Job drawing, mm, ordinate dimensions from the low corner. One solid piece. Coordinates: 2 decimals unless noted, no trailing zeros. Loops run counter-clockwise (first coordinate to the right, second up) from the corner with the lowest first, then second, coordinate; pieces in that order, holes last. Notation, with made-up numbers: (57, 84.5) -> (109, 84.5) arc R32 cw to (109, 123.5) -> close; hole circle Ø1 at (-17.5, 80.25). An arc over 180 degrees is marked (long way). Answer as CSV lines item,"result". Start each with the question number.
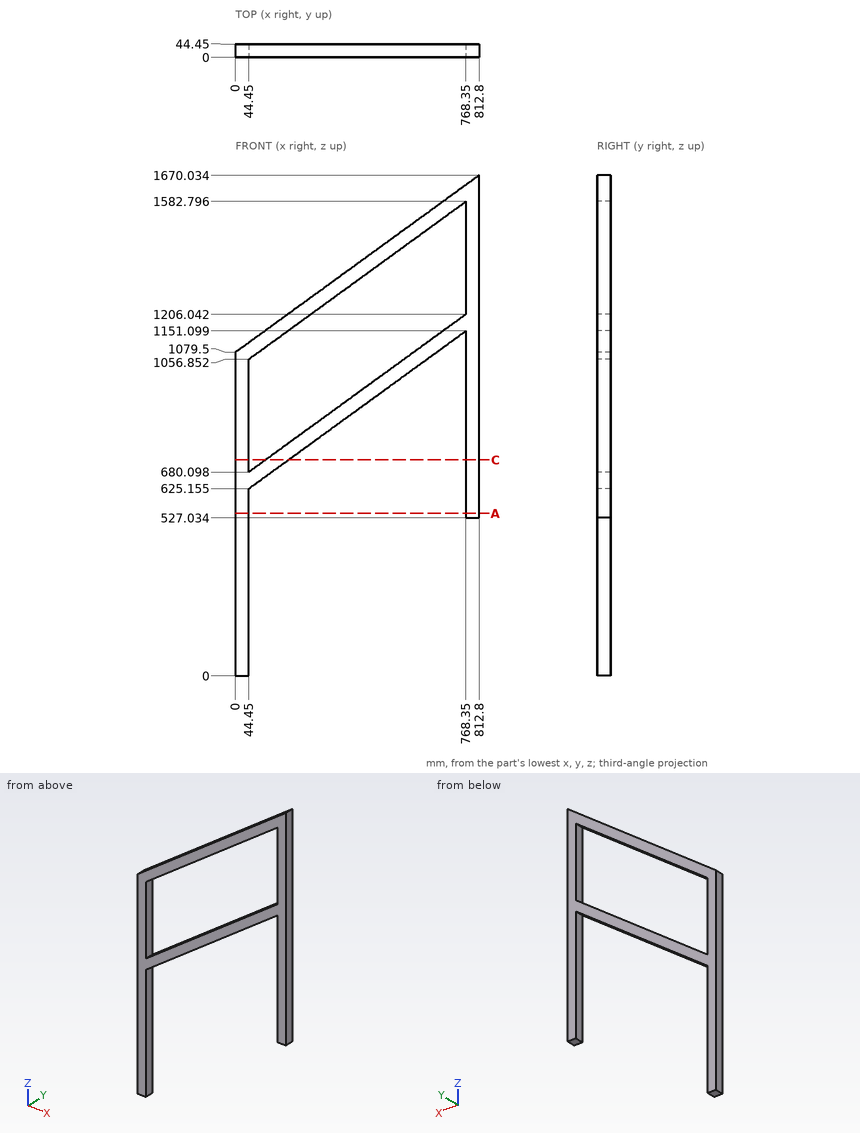
Q1. Saw through at C-C (z = 721). List the corners of the cut face in (x, y), and give its area (3 significant figures).
Q2. Probe probe 1 along X at (y, z) = (19.5, 850.5); probe 2 along X at (y, z) = (21.5, 1107.5); probe 3 along Z at (x, y) = (278, 36.5) (1 decimal). List the from-to ranges inside material, lowest first. Write a range as from..to.
Q3. Pin check, flat tips, straight feed: pin 1 Ø5 at (y, z) = (36.5, 326) entering from +X; pin 2 Ø4 at (x, y) = (359, 39) entering from -Z (1 decimal); pin 3 Ø6 at (x, y) = (556.5, 37.5) entering from -Z. Stop position of each tip, or through.
Q4. Saw through at A-A (z = 542.5). List the corners of the cut face in (x, y), and give its area (3 significant figures).
Ans:
1,outline,"(0, 0) -> (44.45, 0) -> (44.45, 44.45) -> (0, 44.45) -> close; (100.75, 0) -> (176.37, 0) -> (176.37, 44.45) -> (100.75, 44.45) -> close; (768.35, 0) -> (812.8, 0) -> (812.8, 44.45) -> (768.35, 44.45) -> close"
1,area,"7,310 mm²"
2,probe 1,"x = 0..44.45, 278.99..354.61, 768.35..812.8"
2,probe 2,"x = 38.54..114.16, 632.72..708.34, 768.35..812.8"
2,probe 3,"z = 794.8..849.8, 1226.5..1281.5"
3,pin 1,"stops at x = 44.45"
3,pin 2,"stops at z = 852.2"
3,pin 3,"stops at z = 995"
4,outline,"(0, 0) -> (44.45, 0) -> (44.45, 44.45) -> (0, 44.45) -> close; (768.35, 0) -> (812.8, 0) -> (812.8, 44.45) -> (768.35, 44.45) -> close"
4,area,"3,950 mm²"
